```python
from build123d import *

# Parameters (mm, degrees)
F0_R     = 1.5875
F0_R_2   = 1.190625
F1_DEPTH = 3.175
F3_DEPTH = 25.4
F4_DEPTH = 25.4
F5_DEPTH = 25.4
F6_DEPTH = 25.4
F8_DEPTH = 25.4
F9_DEPTH = 21.59
F11_D    = 1.016


with BuildPart() as f1:
    # F0 (on Front) → F1 (new body)
    with BuildSketch(Plane.XZ):
        with BuildLine():
            Line((-59.9854774773, 36.1856259406), (-16.1655526608, 36.1856259406))
            Line((-16.1655526608, 36.1856259406), (-14.5380130693, 39.3606259406))
            Line((-14.5380130693, 39.3606259406), (-16.1655526608, 42.5356259406))
            Line((-16.1655526608, 42.5356259406), (-59.9854774773, 42.5356259406))
            ThreePointArc((-59.9854774773, 42.5356259406), (-63.0682841445, 39.3606259406), (-59.9854774773, 36.1856259406))
        make_face()
        with Locations((-17.3478871584, 39.3606259406)):
            Circle(F0_R, mode=Mode.SUBTRACT)
        with Locations((-17.3478871584, 39.3606259406)):
            Circle(F0_R)
        with Locations((-17.3478871584, 39.3606259406)):
            Circle(F0_R_2, mode=Mode.SUBTRACT)
    extrude(amount=F1_DEPTH)

    # F2 (on face) → F3 (cut)
    with BuildSketch(Plane.XZ.offset(3.175)):
        with BuildLine():
            ThreePointArc((-15.3748723059, 37.758994363), (-16.1969030784, 36.7786361584), (-17.3305589706, 36.1856259406))
            Line((-17.3305589706, 36.1856259406), (-16.1655526608, 36.1856259406))
            Line((-16.1655526608, 36.1856259406), (-15.3517828651, 37.7731259406))
            ThreePointArc((-15.3517828651, 37.7731259406), (-15.3633231409, 37.7660528898), (-15.3748723059, 37.758994363))
        make_face()
        with BuildLine():
            ThreePointArc((-15.404339903, 40.9815081352), (-14.9683940419, 39.3741029339), (-15.3748723059, 37.758994363))
            ThreePointArc((-15.3748723059, 37.758994363), (-15.3633231409, 37.7660528898), (-15.3517828651, 37.7731259406))
            Line((-15.3517828651, 37.7731259406), (-14.5380130693, 39.3606259406))
            Line((-14.5380130693, 39.3606259406), (-15.3517828651, 40.9481259406))
            ThreePointArc((-15.3517828651, 40.9481259406), (-15.3780357265, 40.9648574331), (-15.404339903, 40.9815081352))
        make_face()
        with BuildLine():
            ThreePointArc((-17.4520071596, 42.5356259406), (-16.2702339986, 41.9666642674), (-15.404339903, 40.9815081352))
            ThreePointArc((-15.404339903, 40.9815081352), (-15.3780357265, 40.9648574331), (-15.3517828651, 40.9481259406))
            Line((-15.3517828651, 40.9481259406), (-16.1655526608, 42.5356259406))
            Line((-16.1655526608, 42.5356259406), (-17.4520071596, 42.5356259406))
        make_face()
    extrude(amount=-F3_DEPTH, mode=Mode.SUBTRACT)

    # F2 (on face) → F4 (cut)
    with BuildSketch(Plane.XZ.offset(3.175)):
        with BuildLine():
            ThreePointArc((-20.4132606166, 42.5356259406), (-17.8064403349, 42.0884730118), (-15.404339903, 40.9815081352))
            ThreePointArc((-15.404339903, 40.9815081352), (-16.2702339986, 41.9666642674), (-17.4520071596, 42.5356259406))
            Line((-17.4520071596, 42.5356259406), (-20.4132606166, 42.5356259406))
        make_face()
        with BuildLine():
            ThreePointArc((-15.404339903, 40.9815081352), (-14.9683940419, 39.3741029339), (-15.3748723059, 37.758994363))
            ThreePointArc((-15.3748723059, 37.758994363), (-15.3633231409, 37.7660528898), (-15.3517828651, 37.7731259406))
            Line((-15.3517828651, 37.7731259406), (-14.5380130693, 39.3606259406))
            Line((-14.5380130693, 39.3606259406), (-15.3517828651, 40.9481259406))
            ThreePointArc((-15.3517828651, 40.9481259406), (-15.3780357265, 40.9648574331), (-15.404339903, 40.9815081352))
        make_face()
        with BuildLine():
            Line((-20.778906084, 36.1856259406), (-17.3305589706, 36.1856259406))
            ThreePointArc((-17.3305589706, 36.1856259406), (-16.1969030784, 36.7786361584), (-15.3748723059, 37.758994363))
            ThreePointArc((-15.3748723059, 37.758994363), (-17.9721795073, 36.6126647687), (-20.778906084, 36.1856259406))
        make_face()
    extrude(amount=-F4_DEPTH, mode=Mode.SUBTRACT)

    # F2 (on face) → F5 (cut)
    with BuildSketch(Plane.XZ.offset(3.175)):
        with BuildLine():
            Line((-59.9854774773, 36.1856259406), (-52.4438694119, 36.1856259406))
            ThreePointArc((-52.4438694119, 36.1856259406), (-53.8950663244, 36.5980321526), (-54.9923407048, 37.6334259406))
            Line((-54.9923407048, 37.6334259406), (-59.8919055938, 37.6334259406))
            ThreePointArc((-59.8919055938, 37.6334259406), (-61.6191055938, 39.3606259406), (-59.8919055938, 41.0878259406))
            Line((-59.8919055938, 41.0878259406), (-54.9915987334, 41.0878259406))
            ThreePointArc((-54.9915987334, 41.0878259406), (-53.878578845, 42.1313762088), (-52.4073913693, 42.5356259406))
            Line((-52.4073913693, 42.5356259406), (-59.9854774773, 42.5356259406))
            ThreePointArc((-59.9854774773, 42.5356259406), (-63.0682841445, 39.3606259406), (-59.9854774773, 36.1856259406))
        make_face()
        with BuildLine():
            Line((-58.1647055938, 39.3606259406), (-55.5025643281, 39.3606259406))
            ThreePointArc((-55.5025643281, 39.3606259406), (-55.372064535, 40.261200243), (-54.9915987334, 41.0878259406))
            Line((-54.9915987334, 41.0878259406), (-59.8919055938, 41.0878259406))
            ThreePointArc((-59.8919055938, 41.0878259406), (-58.6705907614, 40.581940773), (-58.1647055938, 39.3606259406))
        make_face()
        with BuildLine():
            Line((-59.8919055938, 37.6334259406), (-54.9923407048, 37.6334259406))
            ThreePointArc((-54.9923407048, 37.6334259406), (-55.3724203009, 38.4601098244), (-55.5025643281, 39.3606259406))
            Line((-55.5025643281, 39.3606259406), (-58.1647055938, 39.3606259406))
            ThreePointArc((-58.1647055938, 39.3606259406), (-58.6705907614, 38.1393111081), (-59.8919055938, 37.6334259406))
        make_face()
        with BuildLine():
            ThreePointArc((-59.8919055938, 41.0878259406), (-61.6191055938, 39.3606259406), (-59.8919055938, 37.6334259406))
            ThreePointArc((-59.8919055938, 37.6334259406), (-58.6705907614, 38.1393111081), (-58.1647055938, 39.3606259406))
            ThreePointArc((-58.1647055938, 39.3606259406), (-58.6705907614, 40.581940773), (-59.8919055938, 41.0878259406))
        make_face()
    extrude(amount=-F5_DEPTH, mode=Mode.SUBTRACT)

    # F2 (on face) → F6 (cut)
    with BuildSketch(Plane.XZ.offset(3.175)):
        with BuildLine():
            ThreePointArc((-52.2927604616, 41.0878259406), (-53.5069291888, 40.578005841), (-54.0090331721, 39.3606259406))
            Line((-54.0090331721, 39.3606259406), (-36.2191055938, 39.3606259406))
            ThreePointArc((-36.2191055938, 39.3606259406), (-35.7132204263, 40.581940773), (-34.4919055938, 41.0878259406))
            Line((-34.4919055938, 41.0878259406), (-52.2927604616, 41.0878259406))
        make_face()
        with BuildLine():
            ThreePointArc((-54.0090331721, 39.3606259406), (-53.5187568392, 38.1547311322), (-52.3259475214, 37.6334259406))
            Line((-52.3259475214, 37.6334259406), (-34.4919055938, 37.6334259406))
            ThreePointArc((-34.4919055938, 37.6334259406), (-35.7132204263, 38.1393111081), (-36.2191055938, 39.3606259406))
            Line((-36.2191055938, 39.3606259406), (-54.0090331721, 39.3606259406))
        make_face()
        with BuildLine():
            ThreePointArc((-34.4919055938, 41.0878259406), (-35.7132204263, 40.581940773), (-36.2191055938, 39.3606259406))
            Line((-36.2191055938, 39.3606259406), (-34.4919055938, 39.3606259406))
            Line((-34.4919055938, 39.3606259406), (-34.4919055938, 41.0878259406))
        make_face()
        with BuildLine():
            ThreePointArc((-36.2191055938, 39.3606259406), (-35.7132204263, 38.1393111081), (-34.4919055938, 37.6334259406))
            Line((-34.4919055938, 37.6334259406), (-34.4919055938, 39.3606259406))
            Line((-34.4919055938, 39.3606259406), (-36.2191055938, 39.3606259406))
        make_face()
        with BuildLine():
            Line((-34.4919055938, 39.3606259406), (-34.4919055938, 37.6334259406))
            ThreePointArc((-34.4919055938, 37.6334259406), (-33.2705907614, 38.1393111081), (-32.7647055938, 39.3606259406))
            ThreePointArc((-32.7647055938, 39.3606259406), (-33.2705907614, 40.581940773), (-34.4919055938, 41.0878259406))
            Line((-34.4919055938, 41.0878259406), (-34.4919055938, 39.3606259406))
        make_face()
    extrude(amount=-F6_DEPTH, mode=Mode.SUBTRACT)

    # F7 (on face) → F8 (cut)
    with BuildSketch(Plane.XZ.offset(3.175)):
        with BuildLine():
            ThreePointArc((-15.6042189064, 38.4623412006), (-15.8016195139, 37.8900751539), (-16.0912083493, 37.3584796926))
            ThreePointArc((-16.0912083493, 37.3584796926), (-15.7292199643, 37.5519041597), (-15.3748723059, 37.758994363))
            ThreePointArc((-15.3748723059, 37.758994363), (-15.1042820518, 38.4073926685), (-14.9774259999, 39.0984404167))
            ThreePointArc((-14.9774259999, 39.0984404167), (-15.285118653, 38.7747704567), (-15.6042189064, 38.4623412006))
        make_face()
        with BuildLine():
            ThreePointArc((-15.6138083064, 40.2906739685), (-15.4922450078, 39.3771200227), (-15.6042189064, 38.4623412006))
            ThreePointArc((-15.6042189064, 38.4623412006), (-15.285118653, 38.7747704567), (-14.9774259999, 39.0984404167))
            ThreePointArc((-14.9774259999, 39.0984404167), (-14.9684104497, 39.3758467508), (-14.9827910636, 39.6530267506))
            ThreePointArc((-14.9827910636, 39.6530267506), (-15.2926534564, 39.9774378811), (-15.6138083064, 40.2906739685))
        make_face()
        with BuildLine():
            ThreePointArc((-16.1121669082, 41.3890946918), (-15.8171331409, 40.8606887152), (-15.6138083064, 40.2906739685))
            ThreePointArc((-15.6138083064, 40.2906739685), (-15.2926534564, 39.9774378811), (-14.9827910636, 39.6530267506))
            ThreePointArc((-14.9827910636, 39.6530267506), (-15.1224646144, 40.3398289098), (-15.404339903, 40.9815081352))
            ThreePointArc((-15.404339903, 40.9815081352), (-15.7541421045, 41.1924412219), (-16.1121669082, 41.3890946918))
        make_face()
    extrude(amount=-F8_DEPTH, mode=Mode.SUBTRACT)

    # F7 (on face) → F9 (cut)
    with BuildSketch(Plane.XZ.offset(3.175)):
        with BuildLine():
            ThreePointArc((-18.3094374963, 42.23041588), (-16.8977827327, 41.3492626146), (-15.6138083064, 40.2906739685))
            ThreePointArc((-15.6138083064, 40.2906739685), (-15.8171331409, 40.8606887152), (-16.1121669082, 41.3890946918))
            ThreePointArc((-16.1121669082, 41.3890946918), (-17.1862834694, 41.8737906284), (-18.3094374963, 42.23041588))
        make_face()
        with BuildLine():
            ThreePointArc((-18.3068840907, 36.5210452642), (-17.1759299722, 36.8786017382), (-16.0912083493, 37.3584796926))
            ThreePointArc((-16.0912083493, 37.3584796926), (-15.8016195139, 37.8900751539), (-15.6042189064, 38.4623412006))
            ThreePointArc((-15.6042189064, 38.4623412006), (-16.8904167196, 37.4010128286), (-18.3068840907, 36.5210452642))
        make_face()
    extrude(amount=-F9_DEPTH, mode=Mode.SUBTRACT)

    # F11 (through all)
    with Locations(Plane(origin=(0, 0, 0), x_dir=(1, 0, 0), z_dir=(0, 1, 0))):
        with Locations((-23.7026810646, -39.3577963114)):
            Hole(F11_D / 2)


solid = f1.part
```
Work out the finished part from the listing and answer in its coordinate system (mm). A direction names the side the tool comes from. Coordinates: 2 decimals unless noted, no trailing zeros. Loops run counter-clockwise (first coordinate to the right, second up) from the corner with the lowest first, then second, coordinate; pieces in that order, holes last. Notation, with made-up numbers: M 28,86.25 L 47,86.25 A10 cw 47,92.25 Z; hole C -23.5,-5.5 d6. An arc over 180 degrees is marked long. Use CSV: the item, a comma, the result in double quotes. Start each with the question number.
(1) Find section A-A, the plane x = -42. Give the vertices of the cut face in (y, z) (3 decimals), then the cut area to 3 significant figures.
(2) For faces 1 (the face through (-36, -2, 42.536)), 2 (the face through (-44, -2, 37.633)), determine the directions among +Z, -Z, +X, -X, +Y, -Y from which every point of the face is accessible in a straight line to the end or side of a thin tool.
(3) Consider line 1 (Z direction, x = -40, y = -0.45); line 2 (X direction, y = -1, z = 38.5); line 3 (X direction, y = -0.4, z = 39). Determine where each line is inside the solid, lowest interval first.
(4) Find section B-B, the plane y = -2.25. Give the vertices of the cut face in (x, z) (1 decimal), then the cut area to 3 significant figures.
(5) For a pull along X with two mould halves and no side action, classify faces 3 (the face through (-16.917, -1.61, 41.363)), 4 (the face through (-31, -3.175, 39)), 5 (the face through (-18.293, -1.565, 38.636)) as +X half, -X half, draft (parallel to the pull), parting line (faces both ways), or undercut.
Recorded:
1,outline,"M -3.175,36.186 L 0,36.186 L 0,37.633 L -3.175,37.633 Z; M -3.175,41.088 L 0,41.088 L 0,42.536 L -3.175,42.536 Z"
1,area,"9.19 mm^2"
2,face 1,"+Z, +X, -X, +Y, -Y"
2,face 2,"+Y, -Y"
3,line 1,"z = 36.19 to 37.63, 41.09 to 42.54"
3,line 2,"x = -55.38 to -53.78, -32.99 to -18.17, -16.53 to -15.59"
3,line 3,"x = -55.48 to -53.97, -32.8 to -24.06, -23.34 to -18.48, -16.21 to -15.51"
4,outline,"M -52.4,36.2 L -20.8,36.2 A10.8 ccw -18.3,36.5 A12.5 ccw -15.6,38.5 A3.6 ccw -15.6,40.3 A12.7 ccw -18.3,42.2 A10.1 ccw -20.4,42.5 L -52.4,42.5 A3.2 ccw Z; hole M -52.3,37.6 L -34.5,37.6 A1.7 ccw -34.5,41.1 L -52.3,41.1 A1.7 ccw Z; hole C -23.7,39.4 d1; hole C -17.3,39.4 d2.4"
4,area,"166 mm^2"
5,face 3,"+X half"
5,face 4,"draft"
5,face 5,"undercut"
